```python
from build123d import *


with BuildPart() as f1:
    # F0 (on Right) → F1 (revolve)
    with BuildSketch(Plane.YZ):
        with BuildLine():
            Line((3.8450945151, 3.429), (2.9765625, 3.429))
            Line((2.9765625, 3.429), (2.9765625, 2.2225))
            ThreePointArc((2.9765625, 2.2225), (2.7905753061, 1.7734871939), (2.3415625, 1.5875))
            Line((2.3415625, 1.5875), (0.4365625, 1.5875))
            ThreePointArc((0.4365625, 1.5875), (0.0058845461, 1.755872204), (-0.1964022384, 2.1717))
            Line((-0.1964022384, 2.1717), (-5.7546875, 2.1717))
            Line((-5.7546875, 2.1717), (-6.5484375, 1.37795))
            Line((-6.5484375, 1.37795), (-6.5484375, 0))
            Line((-6.5484375, 0), (6.5484375, 0))
            Line((6.5484375, 0), (6.9453125, 0))
            ThreePointArc((6.9453125, 0), (6.8848918789, 0.3037549744), (6.7128285076, 0.5612660076))
            Line((6.7128285076, 0.5612660076), (3.8450945151, 3.429))
        make_face()
    revolve(axis=Axis((0, 0.1984375, 0), (0, 1, 0)))


solid = f1.part
```
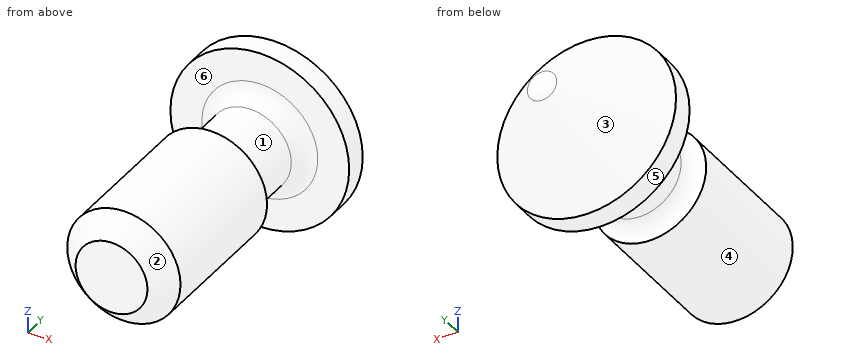
Can you work these out from the model? Positions are in its coordinate system, mm. Face numbers are marked on the shaded views. A direction names the side the tool comes from. Round coordinates to 2 decimals unless told otherwise and drop trailing zeros. Order: outer loops, then holes, each group sorted by start corner. A loop starts at its lowest first (then second) coordinate and runs counter-clockwise, first axis right, second up.
(1) We'd pull the mould along Y, two halves only. Please class the marked faces 1, 2, 3 and 4: +Y half, -Y half, draft (parallel to the pull), parting line (faces both ways), or undercut.
Results are:
face 1: undercut
face 2: -Y half
face 3: +Y half
face 4: draft
(2) If we section it at C-C (y = -5.25): Please give me the cut outline in (x, z).
Results are:
outline: circle Ø4.34 at (0, 0)
(3) If I drill on L1, parallel to Y at x = -1, z = -1.5; L2, parallel to Y at x = 2, z = 0; L3, parallel to Y at x = 1, z = 0.75, over which ranges is the centre line in solid material (lowest first)?
Results are:
L1: y = -6.12 to -0.04, 2.82 to 5.47
L2: y = -5.93 to -0.16, 2.94 to 5.27
L3: y = -6.55 to 6.02
(4) On a 3-axis mill with a long thin cutter (end or side, diameter ignored), from which of +Z, -Z, +X, -X, +Y, -Y can I reach the whole of each face in a straight line? I mean the marked faces 5 and 6. Say none if no direction works.
Results are:
face 5: +Y, -Y
face 6: -Y
(5) I'm going to push flat-ended pins straight in: pin 1 (4 mm diameter, centred on y = -5, z = -1.5, fed in from +X); pin 2 (2 mm diameter, centred on x = -1.5, z = 0.5, fed in from +Y); pin 3 (1.5 mm diameter, centred on x = -1.5, y = 0, fed in from -Z). Where does each tip first touch, or does it pass through?
Results are:
pin 1: stops at x = 2.17
pin 2: stops at y = 6.69
pin 3: stops at z = -2.03
(6) If we section it at B-B (x = 0): Please give me the cut outline in (y, z) (1 decimal), plus the area to 3 significant figures.
Results are:
outline: (-6.5, -1.4) - (-5.8, -2.2) - (-0.2, -2.2) arc R0.6 cw to (0.4, -1.6) - (2.3, -1.6) arc R0.6 cw to (3, -2.2) - (3, -3.4) - (3.8, -3.4) - (6.7, -0.6) arc R0.8 ccw to (6.7, 0.6) - (3.8, 3.4) - (3, 3.4) - (3, 2.2) arc R0.6 cw to (2.3, 1.6) - (0.4, 1.6) arc R0.6 cw to (-0.2, 2.2) - (-5.8, 2.2) - (-6.5, 1.4) - close
area: 55.0 mm2
(7) If we section it at A-A (z = 0): Please give me the cut outline in (x, y) (1 decimal).
Results are:
outline: (-3.4, 3) - (-2.2, 3) arc R0.6 cw to (-1.6, 2.3) - (-1.6, 0.4) arc R0.6 cw to (-2.2, -0.2) - (-2.2, -5.8) - (-1.4, -6.5) - (1.4, -6.5) - (2.2, -5.8) - (2.2, -0.2) arc R0.6 cw to (1.6, 0.4) - (1.6, 2.3) arc R0.6 cw to (2.2, 3) - (3.4, 3) - (3.4, 3.8) - (0.6, 6.7) arc R0.8 ccw to (-0.6, 6.7) - (-3.4, 3.8) - close
(8) If we section it at D-D (y = 5.25): Please give me the cut outline in (x, z), plus the area to 3 significant figures.
Results are:
outline: circle Ø4.05 at (0, 0)
area: 12.9 mm2
